Input: dimensioned drawing with shaded views. Units: mm. Origin: part minimum x, y, z. Give positions to 0.01 mm unless a question says otherwise; leave off trailing zeros. Loops run counter-clockwise (first coordinate to the right, second up) from the corner with the lowest first, then second, coordinate; pieces in that order, holes last.
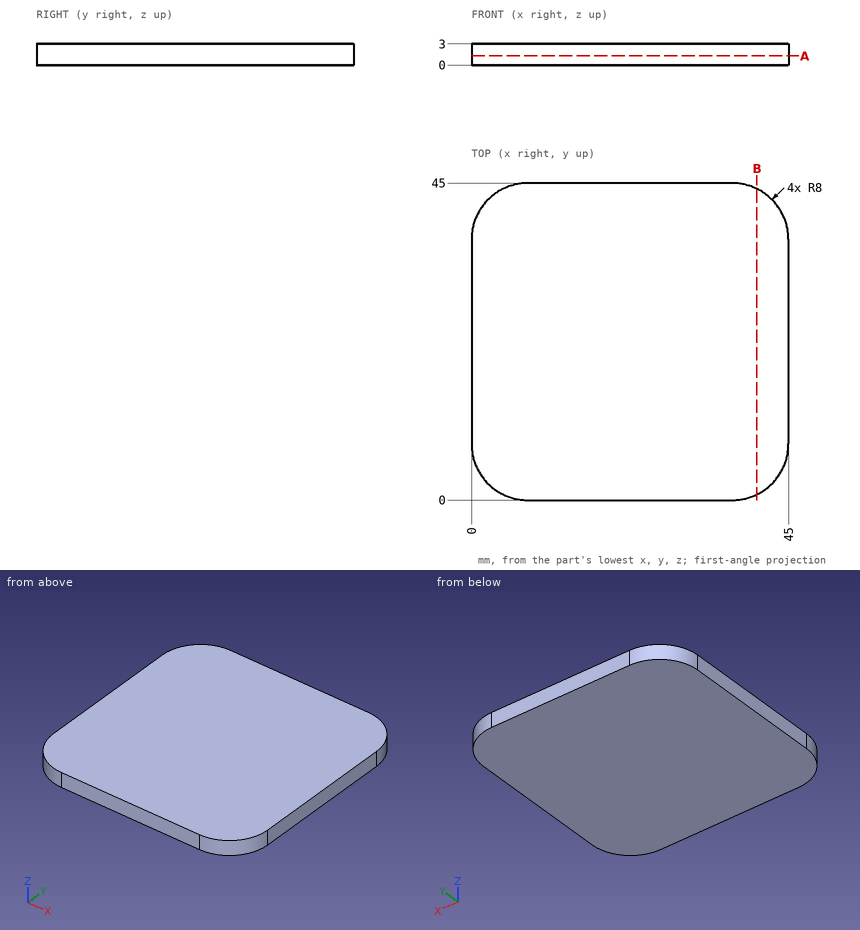
Item 1: Ray query, probe 1 along X at (y, z) = (7, 2.7); probe 2 along Y at (x, z) = (41.5, 0.45); probe 3 along Y at (x, z) = (40.5, 0.8). Return the intervals inside material, ascending.
Values follow:
probe 1: x = 0.06 to 44.94
probe 2: y = 1.39 to 43.61
probe 3: y = 0.81 to 44.19
Item 2: Section query A-A on z = 1.3. Return loops of the section in (x, y), plus the area to 3 significant figures.
Values follow:
outline: (0, 8) arc R8 ccw to (8, 0) - (37, 0) arc R8 ccw to (45, 8) - (45, 37) arc R8 ccw to (37, 45) - (8, 45) arc R8 ccw to (0, 37) - close
area: 1,970 mm2
Item 3: Section query B-B on x = 40.5. Return loops of the section in (y, z).
Values follow:
outline: (0.81, 0) - (44.19, 0) - (44.19, 3) - (0.81, 3) - close
